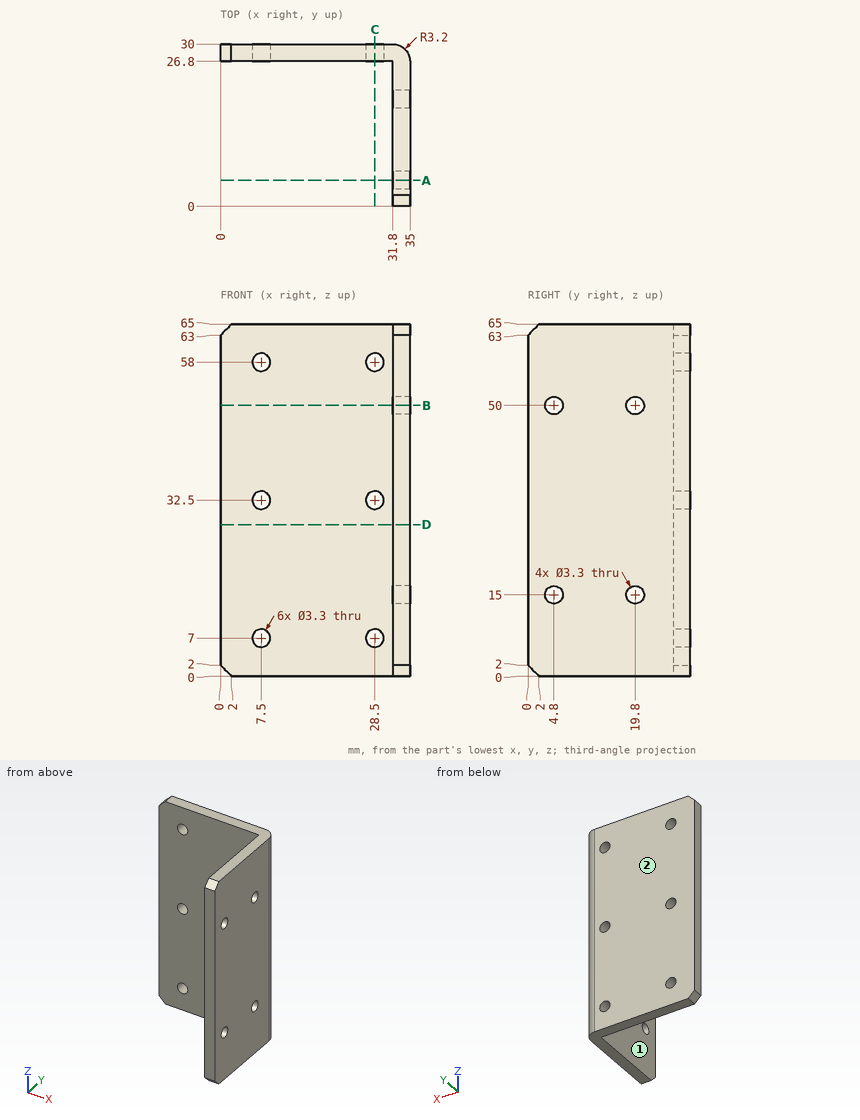
The figure shows three views and two pictorial views of one solid part (mm, origin at its lowest corner). Answer the questions. A direction names the side the tool comes from. Coordinates: 2 decimals unless noted, no trailing zeros. Loops run counter-clockwise (first coordinate to the right, second up) from the corner with the lowest first, then second, coordinate; pieces in that order, holes last.
1) Find section A-A on y = 4.8. Write down the section's boundary in (x, z), then the cut area to 3 significant figures.
2) A tool of negligible diameter and unlimited length cuts with its end or side. For the marked faces 1 and 2, from which of +Z, -Z, +X, -X, +Y, -Y can it reach the whole face along a straight path? Write none if from no direction.
3) Flat-ended cylindrical pins translate along their axes: pin 1 Ø2 at (x, z) = (7.5, 7) entering from +Y; pin 2 Ø4.5 at (x, z) = (28.5, 58) entering from -Y; pin 3 Ø12 at (y, z) = (10.5, 23.5) entering from -X. Find the tip coordinate at first contact, or state that the pin passes through.
4) Find the intervals of material crossed by L1, parallel to Z at x = 28.5, y = 29.3; L2, parallel to Y at x = 32, z = 50; L3, parallel to Y at x = 32.9, z = 15 (3 decimals), in increasing order.
5) Find section B-B on z = 50. Write down the section's boundary in (x, y), then the cut area to 3 significant figures.
6) Find section C-C on x = 28.5. Write down the section's boundary in (y, z).
7) Find section D-D on z = 28. Write down the section's boundary in (x, y).
Values:
1. outline: (31.8, 0) - (35, 0) - (35, 13.35) - (31.8, 13.35) - close; (31.8, 16.65) - (35, 16.65) - (35, 48.35) - (31.8, 48.35) - close; (31.8, 51.65) - (35, 51.65) - (35, 65) - (31.8, 65) - close
1. area: 187 mm2
2. face 1: +Z, -Z, -X, -Y
2. face 2: +Z, -Z, +X, -X, +Y
3. pin 1: passes through
3. pin 2: stops at y = 26.8
3. pin 3: stops at x = 31.8
4. L1: z = 0 to 5.35, 8.65 to 30.85, 34.15 to 56.35, 59.65 to 65
4. L2: y = 0 to 3.15, 6.45 to 18.15, 21.45 to 29.99
4. L3: y = 0 to 3.15, 6.45 to 18.15, 21.45 to 29.805
5. outline: (0, 26.8) - (31.8, 26.8) - (31.8, 21.45) - (35, 21.45) - (35, 26.8) arc R3.2 ccw to (31.8, 30) - (0, 30) - close; (31.8, 0) - (35, 0) - (35, 3.15) - (31.8, 3.15) - close; (31.8, 6.45) - (35, 6.45) - (35, 18.15) - (31.8, 18.15) - close
5. area: 174 mm2
6. outline: (26.8, 0) - (30, 0) - (30, 5.35) - (26.8, 5.35) - close; (26.8, 8.65) - (30, 8.65) - (30, 30.85) - (26.8, 30.85) - close; (26.8, 34.15) - (30, 34.15) - (30, 56.35) - (26.8, 56.35) - close; (26.8, 59.65) - (30, 59.65) - (30, 65) - (26.8, 65) - close
7. outline: (0, 26.8) - (31.8, 26.8) - (31.8, 0) - (35, 0) - (35, 26.8) arc R3.2 ccw to (31.8, 30) - (0, 30) - close
